Here's how the part is built. I have some questions about the finished solid (model axes, mm). Face numbers are marked on the shaded views. A direction names the side the tool comes from. Give positions to 0.01 mm unless a question says otherwise; leave off trailing zeros. Write each loop counter-clockwise with the first axis right and the second up, starting at its lowest first coordinate (ties: lowest second). Pieces come first, ordered by that corner, then holes. Notation, with made-up numbers: (-32, -9) -> (18, -9) arc R23 cw to (18, 0) -> close; hole circle Ø9 at (73.5, -37). An arc over 180 degrees is marked (long way). Return JSON: item names as keys, results as strings.
Autodesk Inventor part; units mm, degrees
ref_plane "YZ Plane" through (0, 0, 0) normal (1, 0, 0) x (0, 1, 0)
ref_plane "XZ Plane" through (0, 0, 0) normal (0, 1, 0) x (-1, 0, 0)
ref_plane "XY Plane" through (0, 0, 0) normal (0, 0, 1) x (1, 0, 0)
sketch "Sketch1" plane through (0, 0, 0) normal (0, 0, 1) x (1, 0, 0)
  arc A0 (-1.9978, -1.5) -> (-1.9978, 1.5) centre (0.0022, 0) ccw
  line L0 (2.5022, 0) -> (-1.9978, 0)
  line L1 (-1.9978, 0) -> (-1.9978, 1.5)
  line L2 (-1.9978, 0) -> (-1.9978, -1.5)
  line L3 (0.0022, 0) -> (20.0022, 0)
  line L4 (0.0022, 0) -> (0.0022, -20)
  line L5 (18.0022, -20) -> (-17.9978, -20)
  line L6 (-19.9978, -18) -> (-19.9978, 18)
  line L7 (-17.9978, 20) -> (18.0022, 20)
  line L8 (20.0022, 18) -> (20.0022, -18)
  line L9 (14.4, 14.4) -> (14.4, 20)
  line L10 (20.0022, 14.4) -> (16.0022, 14.4)
  circle A1 centre (14.4, 14.4) radius 1.6022
  circle A2 centre (14.4, -14.4) radius 1.6022
  circle A3 centre (-14.3955, 14.4) radius 1.6022
  circle A4 centre (-14.3955, -14.4) radius 1.6022
  arc A5 (-17.9978, 20) -> (-19.9978, 18) centre (-17.9978, 18) ccw
  arc A6 (20.0022, 18) -> (18.0022, 20) centre (18.0022, 18) ccw
  arc A7 (18.0022, -20) -> (20.0022, -18) centre (18.0022, -18) ccw
  arc A8 (-19.9978, -18) -> (-17.9978, -20) centre (-17.9978, -18) ccw
  point P0 (0, 0)
  point P1 (0.2522, 0)
  point P2 (-1.9978, 0.75)
  point P3 (-19.9978, 20)
  point P4 (-19.9978, -20)
  point P5 (20.0022, 20)
  dimension "d0" = 5
  dimension "d1" = 4.5
  dimension "d21" = 20
  dimension "d22" = 20
  dimension "d23" = 40
  dimension "d24" = 40
  dimension "d25" = 20
  dimension "d26" = 5.6
  dimension "d27" = 4
  dimension "d28" = 2
extrude "Extrusion1" add sketch "Sketch1" along normal blind 25 contours L3 L8 A7 L5 L4 A0 | A0 L1 L2 L4 L5 A8 L6 A5 L7 L9 A1 L10 L8 L3 | L10 A1 L9 L7 A6 L8
sketch "Sketch2" plane through (-19.9978, -18, 0) normal (-1, 0, 0) x (0, 0, 1)
  line L0 (0, 38) -> (25, 38)
  line L1 (0, 38) -> (12.5, 38)
  line L2 (12.5, 38) -> (12.5, 19.625)
  line L3 (12.5, 18) -> (0, 18)
  line L4 (0, 18) -> (0, 38)
  circle A0 centre (12.5, 18) radius 1.625
  dimension "d33" = 3.25
  dimension "d31" = 12.5
  dimension "d32" = 20
extrude "Extrusion2" cut sketch "Sketch2" against normal blind 20 contours A0
sketch "Sketch3" plane through (0, 0, 25) normal (0, 0, 1) x (1, 0, 0)
  line L0 (58, -20) -> (-18, -20)
  line L1 (-20, -18) -> (-20, 18)
  line L2 (-18, 20) -> (58, 20)
  line L3 (60, 18) -> (60, -18)
  arc A0 (58, -20) -> (60, -18) centre (58, -18) ccw
  arc A1 (60, 18) -> (58, 20) centre (58, 18) ccw
  arc A2 (-18, 20) -> (-20, 18) centre (-18, 18) ccw
  arc A3 (-20, -18) -> (-18, -20) centre (-18, -18) ccw
  point P0 (0, 0)
  dimension "d36" = 60
  dimension "d37" = 20
  dimension "d38" = 20
  dimension "d39" = 20
  dimension "d40" = 2
extrude "Extrusion3" add sketch "Sketch3" along normal blind 10
sketch "Sketch7" plane through (0, 0, 35) normal (0, 0, 1) x (1, 0, 0)
  line L0 (55.0022, 20) -> (50.0022, 20)
  line L1 (50.0022, 20) -> (50.0022, 15)
  line L2 (50.0022, 15) -> (55.0022, 15)
  line L3 (55.0022, 15) -> (55.0022, 20)
  circle A0 centre (50.0022, 15) radius 1.6
  line L4 (18.0022, 20) -> (-17.9978, 20)
  line L5 (0.0022, 20) -> (60.0022, 20)
  line L6 (60.0022, 20) -> (60.0022, -20)
  line L7 (60.0022, -20) -> (0.0022, -20)
  line L8 (0.0022, -20) -> (0.0022, 20)
  circle A1 centre (50.0022, -15) radius 1.6
  line L9 (60.0022, -20) -> (20.0022, -20)
  line L10 (20.0022, -20) -> (20.0022, 20)
  line L11 (20.0022, 20) -> (60.0022, 20)
  line L12 (60.0022, 20) -> (60.0022, -20)
  line L13 (58, 20) -> (-18, 20)
  line L14 (40.0022, 20) -> (40.0022, -20)
  circle A2 centre (30.0022, 15) radius 1.6
  circle A3 centre (30.0022, -15) radius 1.6
  point P0 (0, 0)
  dimension "d73" = 5
  dimension "d74" = 5
  dimension "d75" = 3.2
  dimension "d78" = 60
  dimension "d81" = 60
  dimension "d85" = 40
  dimension "d86" = 30
  dimension "d87" = 20
extrude "Extrusion6" cut sketch "Sketch7" against normal blind 20 contours A0 L2 L1 | L1 L2 A0 | A1 | A2 | A3
fillet "Fillet3" radius 2 5 edges at (59.4142, -19.4142, 25) (60, 0, 25) (59.4142, 19.4142, 25) (38.0011, 20, 25) (38.0011, -20, 25)
properties part number "afterdesign"
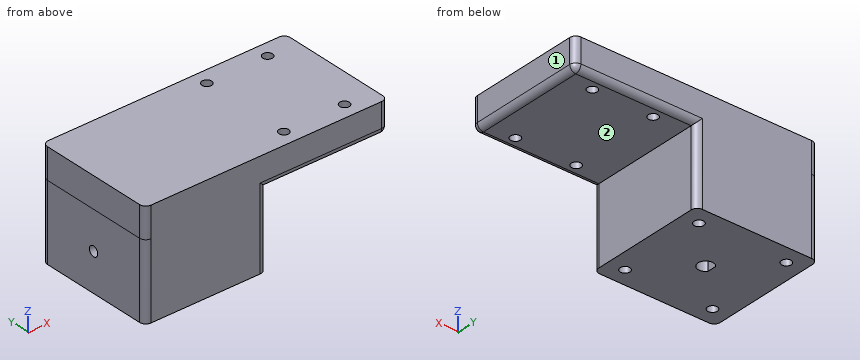
1. If I drill on line 1 (Y direction, x = 14.4, z = 10.75); line 2 (Y direction, x = 13, z = 19.5); line 3 (Z direction, x = 50, y = 2), over which ranges is the centre line in solid material (lowest first)? Write a range as [from, to].
Taken from the geometry:
{"line 1": "y = [-20, -16], [-12.8, 12.8], [16, 20]", "line 2": "y = [-20, -15.18], [-13.62, 13.62], [15.18, 20]", "line 3": "z = [25, 35]"}
2. Suppose I cut it at D-D, the plane x = 24. List the corners of the cut face in (y, z) for me, and give its area (3 significant figures).
Taken from the geometry:
{"outline": "(-20, 27) arc R2 ccw to (-18, 25) -> (18, 25) arc R2 ccw to (20, 27) -> (20, 35) -> (-20, 35) -> close", "area": "398 mm²"}
3. Suppose I cut it at C-C, the plane x = 14.4. List the corners of the cut face in (y, z) for me.
Taken from the geometry:
{"outline": "(-20, 0) -> (-16, 0) -> (-16, 25) -> (-12.8, 25) -> (-12.8, 0) -> (12.8, 0) -> (12.8, 25) -> (16, 25) -> (16, 0) -> (20, 0) -> (20, 35) -> (-20, 35) -> close"}
4. For pin 1 Ø6 at (x, y) = (29.5, -8.5) entering from -Z; pin 2 Ø3.5 at (x, y) = (14.4, 14.4) entering from -Z; pin 3 Ø5 at (y, z) = (0, 12.5) entering from +X; pin 4 Ø8 at (y, z) = (-4.5, 9.5) entering from -X, each with a flat end and sliding along its axis, tell me the tip position at first contact or that it passes through.
Taken from the geometry:
{"pin 1": "stops at z = 25", "pin 2": "stops at z = 0", "pin 3": "stops at x = 20", "pin 4": "stops at x = -20"}
5. Which directions (+Z, -Z, +X, -X, +Y, -Y) give clear straight access to the entire face, cutting with the end or side of a thin tool? Please do the marked faces 1 and 2.
Taken from the geometry:
{"face 1": "+Z, -Z, +X, +Y, -Y", "face 2": "-Z, +X, +Y, -Y"}
